from build123d import *

# Parameters (mm, degrees)
PAD001_DEPTH    = 6
CLONE2D004_R    = 9
CLONE2D004_R_2  = 4
POCKET004_DEPTH = 6.001
SKETCH009_R     = 27.5
POCKET005_DEPTH = 6.001
SKETCH010_R     = 31
POCKET006_DEPTH = 2


with BuildPart() as part:
    # Clone2D003 → Pad001 (new body)
    with BuildSketch(Plane.XY):
        with BuildLine():
            ThreePointArc((9.526279, 54), (0, 59.5), (-9.526279, 54))
            Line((-9.526279, 54), (-51.528512, -18.75))
            ThreePointArc((-51.528512, -18.75), (-51.528512, -29.75), (-42.002232, -35.25))
            Line((-42.002232, -35.25), (42.002232, -35.25))
            ThreePointArc((42.002232, -35.25), (51.528512, -29.75), (51.528512, -18.75))
            Line((51.528512, -18.75), (9.526279, 54))
        make_face()
    extrude(amount=-PAD001_DEPTH)

    # Clone2D004 → Pocket004 (cut, through all)
    with BuildSketch(Plane.XY):
        with Locations((0, 48.5)):
            Circle(CLONE2D004_R)
        with Locations((-42.002232, -24.25)):
            Circle(CLONE2D004_R)
        with Locations((42.002232, -24.25)):
            Circle(CLONE2D004_R)
        Circle(CLONE2D004_R_2)
    extrude(amount=-POCKET004_DEPTH, mode=Mode.SUBTRACT)

    # Sketch009 → Pocket005 (cut, through all)
    with BuildSketch(Plane.XY):
        Circle(SKETCH009_R)
    extrude(amount=-POCKET005_DEPTH, mode=Mode.SUBTRACT)

    # Sketch010 → Pocket006 (cut)
    with BuildSketch(Plane.XY):
        Circle(SKETCH010_R)
    extrude(amount=-POCKET006_DEPTH, mode=Mode.SUBTRACT)


solid = part.part
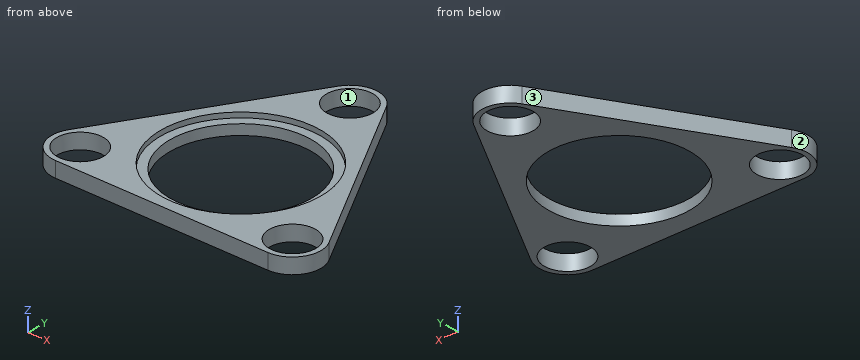
The model under review builds one solid part; all positions refer to its coordinate system, in mm. Face numbers are marked on the shaded views. Coordinates: 2 decimals unless noted, no trailing zeros. Loops run counter-clockwise (first coordinate to the right, second up) from the corner with the lowest first, then second, coordinate; pieces in that order, holes last. Notation, with made-up numbers: (24, 33.5) -> (33, 33.5) arc R19 cw to (33, 54.5) -> close; hole circle Ø5 at (40, 80). An arc over 180 degrees is marked (long way). Use a Markdown table: item, result. Add a question column.
1. Add section D-D on x = -40. Write out the cut boundary in (y, z), plus the area to 3 significant figures.
2. Add section C-C on y = 5.5. Write out the cut boundary in (x, z), plus the area to 3 significant figures.
3. To check wall thickness, follow line 1 (X direction, y = -7, z = -4.75); line 2 (X direction, y = 4, z = -5.65); line 3 (Z direction, x = 16, y = -23). State the ranges of each line that lie inside material, in increasing order.
4. Clearance check with flat-ended pins moving along their axes: pin 1 Ø2 at (y, z) = (12, -3) entering from +X; pin 2 Ø2 at (x, z) = (-24.5, -2.5) entering from +Y; pin 3 Ø8 at (x, y) = (-23.5, 45.5) entering from -Z. State where each tip first meets the part, or that it passes through.
5. Add section B-B on z = -3.4. Write out the cut boundary in (x, y).
6. Add section A-A on x = 0. Write out the cut boundary in (y, z), plus the area to 4 significant figures.
7. Draft analysis for pull direction Y (two halves, no side actions). For the marked faces 1, 2 and 3, state which applies: pulls with the +Y half, pulls with the -Y half, needs draft (parallel to the pull), parting line crosses it, or undercut.
Returned:
| question | item | result |
|---|---|---|
| 1 | outline | (-35.25, -6) -> (-33.02, -6) -> (-33.02, 0) -> (-35.25, 0) -> close; (-15.48, -6) -> (1.22, -6) -> (1.22, 0) -> (-15.48, 0) -> close |
| 1 | area | 114 mm² |
| 2 | outline | (-37.53, -6) -> (-26.94, -6) -> (-26.94, -2) -> (-30.51, -2) -> (-30.51, 0) -> (-37.53, 0) -> close; (26.94, -6) -> (37.53, -6) -> (37.53, 0) -> (30.51, 0) -> (30.51, -2) -> (26.94, -2) -> close |
| 2 | area | 113 mm² |
| 3 | line 1 | x = -44.74 to -26.59, 26.59 to 44.74 |
| 3 | line 2 | x = -38.39 to -27.21, 27.21 to 38.39 |
| 3 | line 3 | z = -6 to -2 |
| 4 | pin 1 | stops at x = 34.35 |
| 4 | pin 2 | stops at y = 29.8 |
| 4 | pin 3 | passes through |
| 5 | outline | (-51.53, -18.75) arc R11 ccw to (-42, -35.25) -> (42, -35.25) arc R11 ccw to (51.53, -18.75) -> (9.53, 54) arc R11 ccw to (-9.53, 54) -> close; hole circle Ø18 at (-42, -24.25); hole circle Ø55 at (0, 0); hole circle Ø18 at (0, 48.5); hole circle Ø18 at (42, -24.25) |
| 6 | outline | (-35.25, -6) -> (-27.5, -6) -> (-27.5, -2) -> (-31, -2) -> (-31, 0) -> (-35.25, 0) -> close; (27.5, -6) -> (39.5, -6) -> (39.5, 0) -> (31, 0) -> (31, -2) -> (27.5, -2) -> close; (57.5, -6) -> (59.5, -6) -> (59.5, 0) -> (57.5, 0) -> close |
| 6 | area | 116.5 mm² |
| 7 | face 1 | undercut |
| 7 | face 2 | parting line crosses it |
| 7 | face 3 | pulls with the +Y half |
